from build123d import *

# Parameters (mm, degrees)
M20X0_5_TAPPED_HOLE1_D     = 19.5
M20X0_5_TAPPED_HOLE1_DEPTH = 54
M20X0_5_TAPPED_HOLE1_TIP   = 5.858391036
CHAMFER1_SIZE              = 5
FILLET3_R                  = 1
CIRPATTERN1_COUNT          = 3


with BuildPart() as part:
    # Sketch1 → Revolve1 (revolve)
    with BuildSketch(Plane(origin=(0, 0, 0), x_dir=(0, 0, -1), z_dir=(1, 0, 0))):
        Polygon((0, 0), (-30, 0), (-30, 30), (-25, 30), (-25, 73), (-27, 74.450346012), (-27, 98), (0, 98), align=None)
    revolve(axis=Axis((0, 214.375507313, 0), (0, -1, 0)))

    # M20x0.5 Tapped Hole1
    with Locations(Plane(origin=(-0.400317765, 98, -0.390314584), x_dir=(0, 0, 1), z_dir=(0, 1, 0))):
        with Locations((0, 0)):
            Hole(M20X0_5_TAPPED_HOLE1_D / 2, depth=M20X0_5_TAPPED_HOLE1_DEPTH)
            with Locations((0, 0, -(M20X0_5_TAPPED_HOLE1_DEPTH + M20X0_5_TAPPED_HOLE1_TIP / 2))):  # 118° drill point
                Cone(0, M20X0_5_TAPPED_HOLE1_D / 2, M20X0_5_TAPPED_HOLE1_TIP, mode=Mode.SUBTRACT)

    # Chamfer1
    chamfer1_edges = [part.edges().sort_by_distance(p)[0] for p in [
        (0, 30, -30),
    ]]
    chamfer(chamfer1_edges, length=CHAMFER1_SIZE - 0.0001)  # a hair under: the kernel refuses the full size

    # Fillet3
    fillet3_edges = [part.edges().sort_by_distance(p)[0] for p in [
        (0, 98, -27),
    ]]
    fillet(fillet3_edges, radius=FILLET3_R)

    # Sketch4 → M6x0.5 Tapped Hole1 (revolve, cut)
    with BuildSketch(Plane(origin=(-0.125783676, 0, 19.999604458), x_dir=(0, 0, -1), z_dir=(1, 0, 0))):
        Polygon((0, 0), (0, 26.652366702), (2.75, 25), (2.75, 0), align=None)
    m6x0_5_tapped_hole1 = revolve(axis=Axis((-0.125783676, -6.35, 19.999604458), (0, 1, 0)), mode=Mode.SUBTRACT)

    # CirPattern1: M6x0.5 Tapped Hole1 ×3 about axis
    cirpattern1_axis = Axis((0.001065889, 0, -0.169476304), (0, 1, 0))
    for i in range(1, CIRPATTERN1_COUNT):
        add(m6x0_5_tapped_hole1.rotate(cirpattern1_axis, i * 360 / CIRPATTERN1_COUNT), mode=Mode.SUBTRACT)


solid = part.part
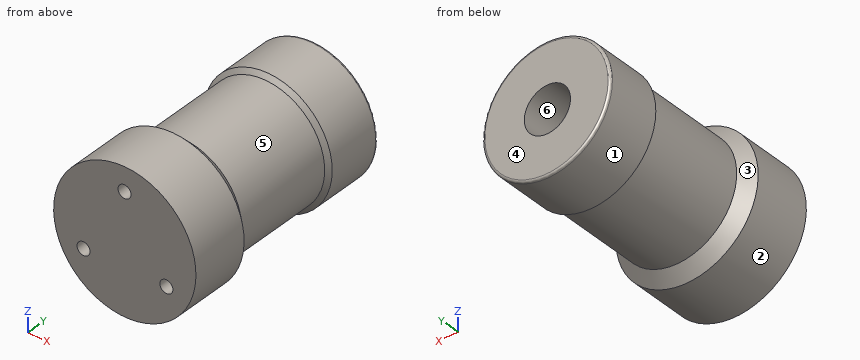
Model file for the job. Use its own axes, mm. Face numbers are marked on the shaded views. A direction names the side the tool comes from. Give positions to 0.01 mm unless a question says otherwise; leave off trailing zeros. Loops run counter-clockwise (first coordinate to the right, second up) from the corner with the lowest first, then second, coordinate; pieces in that order, holes last.
Item 1: Mould opens along Y. For the marked faces 3, 4, 5 and 6 say: +Y half, -Y half, draft (parallel to the pull), parting line (faces both ways), or undercut.
Check values:
face 3: undercut
face 4: +Y half
face 5: undercut
face 6: draft
Item 2: Which spindle directions (+Z, -Z, +X, -X, +Y, -Y) get a long thin tool onto all of the face, cutting with end or side? Do the marked faces 1 and 2. Say none if no direction does.
Check values:
face 1: +Y
face 2: +Y, -Y
Item 3: Drill centre lines: line 1 along Z through (x, y) = (-5, 46.5); line 2 along Z through (x, y) = (8, 58); line 3 along X through (y, z) = (75, -4). Where is each one in solid material? Low to high.
Check values:
line 1: z = -24.49 to -8.99, 8.21 to 24.49
line 2: z = -23.69 to -5.34, 4.56 to 23.69
line 3: x = -26.7 to -9.46, 8.66 to 26.7
Item 4: Drop flat-ended pins along their axis: P1, Ø2, axis at x = 8.5, y = 79, coming from the -Z side; P2, Ø3, axis at x = 5, y = 17, coming from the -Z side; P3, Ø1.5, axis at x = 6, y = 17.5, coming from the -Z side. Give the stop position or say it passes through.
Check values:
P1: stops at z = -25.94
P2: stops at z = -29.8
P3: stops at z = -29.54
Item 5: Slice it at B-B (y = 13). Write the cut outline in (x, z).
Check values:
outline: circle Ø60 at (0, 0); hole circle Ø5.5 at (-17.4, -10.36); hole circle Ø5.5 at (-0.13, 20); hole circle Ø5.5 at (17.53, -10.14)
Item 6: Slice it at A-A (y = 33.5). Write the cut outline in (x, z).
Check values:
outline: circle Ø50 at (0, 0)
